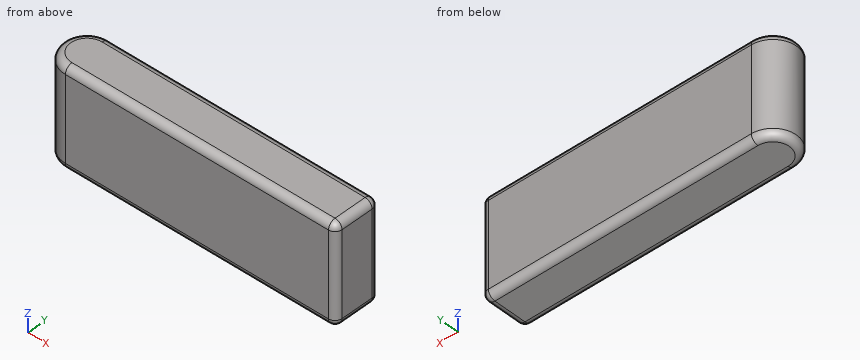
```python
from build123d import *

# Parameters (mm, degrees)
SKETCH1_W           = 104
SKETCH1_H           = 35
BOSS_EXTRUDE1_DEPTH = 16.5
FILLET2_RADIUS      = 8.25
FILLET2_LENGTH      = 35
FILLET3_R           = 2.5


with BuildPart() as part:
    # Sketch1 → Boss-Extrude1 (new body)
    with BuildSketch(Plane(origin=(0, 0, 0), x_dir=(1, 0, 0), z_dir=(0, 1, 0))):
        Rectangle(SKETCH1_W, SKETCH1_H)
    extrude(amount=BOSS_EXTRUDE1_DEPTH)

    # Fillet2: full round fillet: the end face becomes a half cylinder, R = half its width
    fillet2_face = Plane((-52, 8.25, 0), x_dir=(0, 0, -1), z_dir=(-1, 0, 0))  # on the end face: x along it, z out of the body
    fillet2_slab = fillet2_face.offset(-FILLET2_RADIUS / 2) * Box(FILLET2_LENGTH, 2 * FILLET2_RADIUS, FILLET2_RADIUS, mode=Mode.PRIVATE)  # the body's end, R deep
    fillet2_round = Plane((-43.75, 8.25, 0), x_dir=(-1, 0, 0), z_dir=(0, 0, -1)) * Cylinder(FILLET2_RADIUS, FILLET2_LENGTH, mode=Mode.PRIVATE)  # its axis R under the face
    add(fillet2_slab - fillet2_round, mode=Mode.SUBTRACT)

    # Fillet3
    fillet3_edges = [part.edges().sort_by_distance(p)[0] for p in [
        (52, 16.5, 0),
        (4.125, 16.5, 17.5),
        (4.125, 0, 17.5),
        (4.125, 16.5, -17.5),
        (-52, 8.25, -17.5),
        (-52, 8.25, 17.5),
        (4.125, 0, -17.5),
        (52, 0, 0),
        (52, 8.25, -17.5),
        (52, 8.25, 17.5),
    ]]
    fillet(fillet3_edges, radius=FILLET3_R)


solid = part.part
```
Geometry check sheet. Reference: the model listing, model coordinates, mm. Round coordinates to 2 decimals unless told otherwise and drop trailing zeros. Loops run counter-clockwise (first coordinate to the right, second up) from the corner with the lowest first, then second, coordinate; pieces in that order, holes last. Notation, with made-up numbers: (82.25, -29.5) - (114.25, -29.5) arc R32 cw to (114.25, -3.5) - close; hole circle Ø7 at (73.25, -2.5). An arc over 180 degrees is marked (long way). Write item = value, one per line. Start each with the question number.
1. Thickness scan on line 1 (X direction, y = 1.75, z = 0.5); line 2 (X direction, y = 14.25, z = -8); line 3 (Z direction, x = 39.5, y = 1.75). Record the ranges inside material, lowest first.
2. Depth check by flat-ended pin: pin 1 (3 mm diameter, centred on y = 4.5, z = 6, fed in from -X). Enter the tip coordinate at first touch or a pass-through.
3. Section check A-A on z = -13. Enter the section's corners in (x, y).
Working result:
q1.line_1 = -48.83 to 51.88
q1.line_2 = -49.41 to 51.99
q1.line_3 = -17.38 to 17.38
q2.pin_1 = -51.69
q3.outline = (-43.75, 0) - (49.5, 0) arc R2.5 ccw to (52, 2.5) - (52, 14) arc R2.5 ccw to (49.5, 16.5) - (-43.75, 16.5) arc R8.25 ccw to start
